Model file for the job. Use its own axes, mm. Face numbers are marked on the shaded views. A direction names the side the tool comes from. Round coordinates to 2 decimals unless told otherwise and drop trailing zeros. Loops run counter-clockwise (first coordinate to the right, second up) from the corner with the lowest first, then second, coordinate; pieces in that order, holes last. Notation, with made-up numbers: (65.5, 77.25) -> (85.5, 77.25) arc R16 ccw to (85.5, 104.25) -> close; hole circle Ø11 at (20, 44). An arc over 180 degrees is marked (long way). Use a Markdown table: item, result.
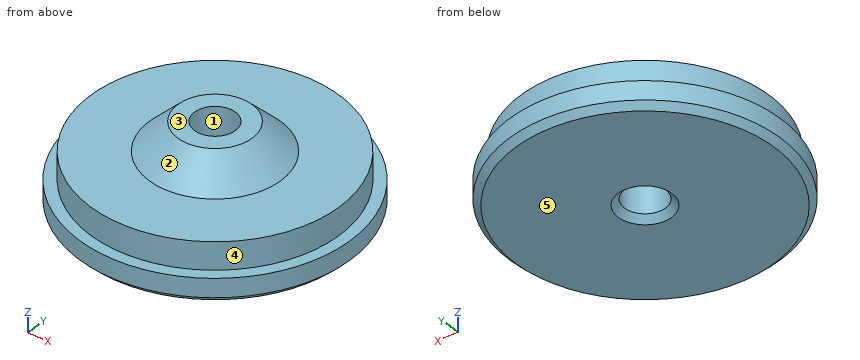
from build123d import *

# Parameters (mm, degrees)
SKETCH1_R           = 10.9
BOSS_EXTRUDE1_DEPTH = 2
SKETCH2_R           = 10
BOSS_EXTRUDE2_DEPTH = 2.2
SKETCH4_R           = 3
BOSS_EXTRUDE3_DEPTH = 2.3
SKETCH3_R           = 1.65
CUT_EXTRUDE1_DEPTH  = 17.729315587
CHAMFER1_SIZE       = 2.3
CHAMFER2_SIZE       = 0.5
CHAMFER3_SIZE       = 0.5


with BuildPart() as part:
    # Sketch1 → Boss-Extrude1 (new body)
    with BuildSketch(Plane.XY):
        Circle(SKETCH1_R)
    extrude(amount=BOSS_EXTRUDE1_DEPTH)

    # Sketch2 → Boss-Extrude2 (add)
    with BuildSketch(Plane.XY.offset(2)):
        Circle(SKETCH2_R)
    extrude(amount=BOSS_EXTRUDE2_DEPTH)

    # Sketch4 → Boss-Extrude3 (add)
    with BuildSketch(Plane.XY.offset(4.2)):
        Circle(SKETCH4_R)
    extrude(amount=BOSS_EXTRUDE3_DEPTH)

    # Sketch3 → Cut-Extrude1 (cut, through all)
    with BuildSketch(Plane(origin=(0, 0, 0), x_dir=(-1, 0, 0), z_dir=(0, 0, -1))):
        Circle(SKETCH3_R)
    extrude(amount=-CUT_EXTRUDE1_DEPTH, mode=Mode.SUBTRACT)

    # Chamfer1
    chamfer1_edges = [part.edges().sort_by_distance(p)[0] for p in [
        (-3, 0, 4.2),
    ]]
    chamfer(chamfer1_edges, length=CHAMFER1_SIZE - 0.0001)  # a hair under: the kernel refuses the full size

    # Chamfer2
    chamfer2_edges = [part.edges().sort_by_distance(p)[0] for p in [
        (1.65, 0, 0),
    ]]
    chamfer(chamfer2_edges, length=CHAMFER2_SIZE)

    # Chamfer3
    chamfer3_edges = [part.edges().sort_by_distance(p)[0] for p in [
        (-10.9, 0, 0),
    ]]
    chamfer(chamfer3_edges, length=CHAMFER3_SIZE)


solid = part.part
Q1. Band-saw the part on D-D, the plane z = 5. Give the cut face in (x, y), plus the area to 3 significant figures.
Results list:
| item | result |
|---|---|
| outline | circle Ø9 at (0, 0); hole circle Ø3.3 at (0, 0) |
| area | 55.1 mm² |
Q2. Pull direction Y, two halves, no side cores. Call the marked faces 1, 2 and 3: released by +Y, released by -Y, zero draft, split by the parting line, or undercut.
Results list:
| item | result |
|---|---|
| face 1 | undercut |
| face 2 | split by the parting line |
| face 3 | zero draft |
Q3. Flat gauge pins, fed straight in: pin 1 (2 mm diameter, centred on x = 8.5, z = 5, fed in from +Y); pin 2 (1.5 mm diameter, centred on y = -1, z = 1, fed in from +X); pin 3 (1 mm diameter, centred on y = 6, z = 4, fed in from -X). Where does each tip first touch, or does it go through?
Results list:
| item | result |
|---|---|
| pin 1 | stops at y = 6.13 |
| pin 2 | stops at x = 10.9 |
| pin 3 | stops at x = -8.35 |
Q4. Drill centre lines: L1, parallel to Y at x = 0, z = 2.1; L2, parallel to Z at x = -5.5, y = -3; L3, parallel to X at y = 0.75, z = 6. Where is each one in solid material? Low to high. Write a range as from..to.
Results list:
| item | result |
|---|---|
| L1 | y = -10..-1.65, 1.65..10 |
| L2 | z = 0..4.2 |
| L3 | x = -3.42..-1.47, 1.47..3.42 |
Q5. Band-saw the part on C-C, the plane z = 2.5. Give the cut face in (x, y).
Results list:
| item | result |
|---|---|
| outline | circle Ø20 at (0, 0); hole circle Ø3.3 at (0, 0) |
Q6. Tool access for the marked faces 4 and 5: list every direction of +Z, -Z, +X, -X, +Y, -Y with a clear straight run to the whole face (end or side of a thin tool).
Results list:
| item | result |
|---|---|
| face 4 | +Z |
| face 5 | -Z, +X, -X, +Y, -Y |
